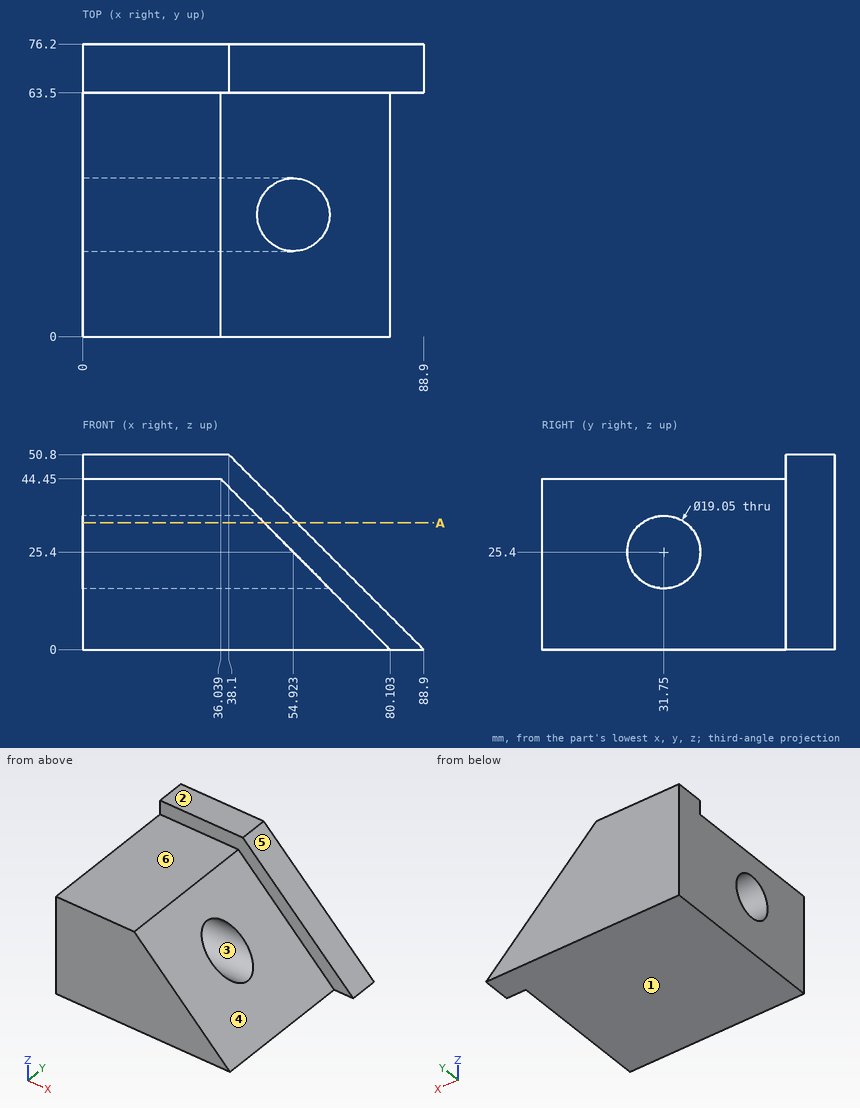
The figure shows three views and two pictorial views of one solid part (mm, origin at its lowest corner). Answer the questions. A direction names the side the tool comes from. Coordinates: 2 decimals unless noted, no trailing zeros. Loops run counter-clockwise (first coordinate to the right, second up) from the corner with the lowest first, then second, coordinate; pieces in that order, holes last. Notation, with made-up numbers: (-16.5, 77) -> (-11.5, 77) arc R36 cw to (-11.5, 112) -> close; hole circle Ø2 at (14, 77.25). An arc over 180 degrees is marked (long way). Write item = value, one per line. Start each with the question number.
1) The mould has two halves that part along Z. Classify the marked faces 1, 2 and 3: released by +Z, released by -Z, zero draft, split by the parting line, or undercut.
2) Given pin 1 Ø1.5 at (y, z) = (61.5, 8) entering from +X (1 decimal); pin 2 Ø17 at (y, z) = (31.75, 25.4) entering from +X; pin 3 Ø11 at (x, y) = (21, 41.5) entering from +Z, each flat-ended and moving along its own axis, determine where each tip first touches the part or whether it passes through.
3) A tool of negligible diameter and unlimited length cuts with its end or side. For the marked faces 4, 5 and 6, from which of +Z, -Z, +X, -X, +Y, -Y can it reach the whole face along a straight path? Write none if from no direction.
4) A cutting plane is placed at A-A (z = 33). Give the vertices of the cut face in (x, y), then the cut area to 4 significant figures.
5) Straight lines are drawn through the part: line 1 (Y direction, x = 42, z = 25); line 2 (Z direction, x = 15.5, y = 9.5); line 3 (Z direction, x = 25, y = 34.5). For each, find the intervals that lie inside material, in ascending order. Write a range as from..to.
Responses:
q1.face_1 = released by -Z
q1.face_2 = released by +Z
q1.face_3 = undercut
q2.pin_1 = 72.9
q2.pin_2 = through
q2.pin_3 = 44.45
q3.face_4 = +Z, +X, -Y
q3.face_5 = +Z, +X, +Y, -Y
q3.face_6 = +Z, +X, -X, -Y
q4.outline = (0, 0) -> (47.39, 0) -> (47.39, 26.01) -> (0, 26.01) -> close; (0, 37.49) -> (47.39, 37.49) -> (47.39, 63.5) -> (55.9, 63.5) -> (55.9, 76.2) -> (0, 76.2) -> close
q4.area = 3,175 mm²
q5.line_1 = 0..22.23, 41.27..76.2
q5.line_2 = 0..44.45
q5.line_3 = 0..16.28, 34.52..44.45
